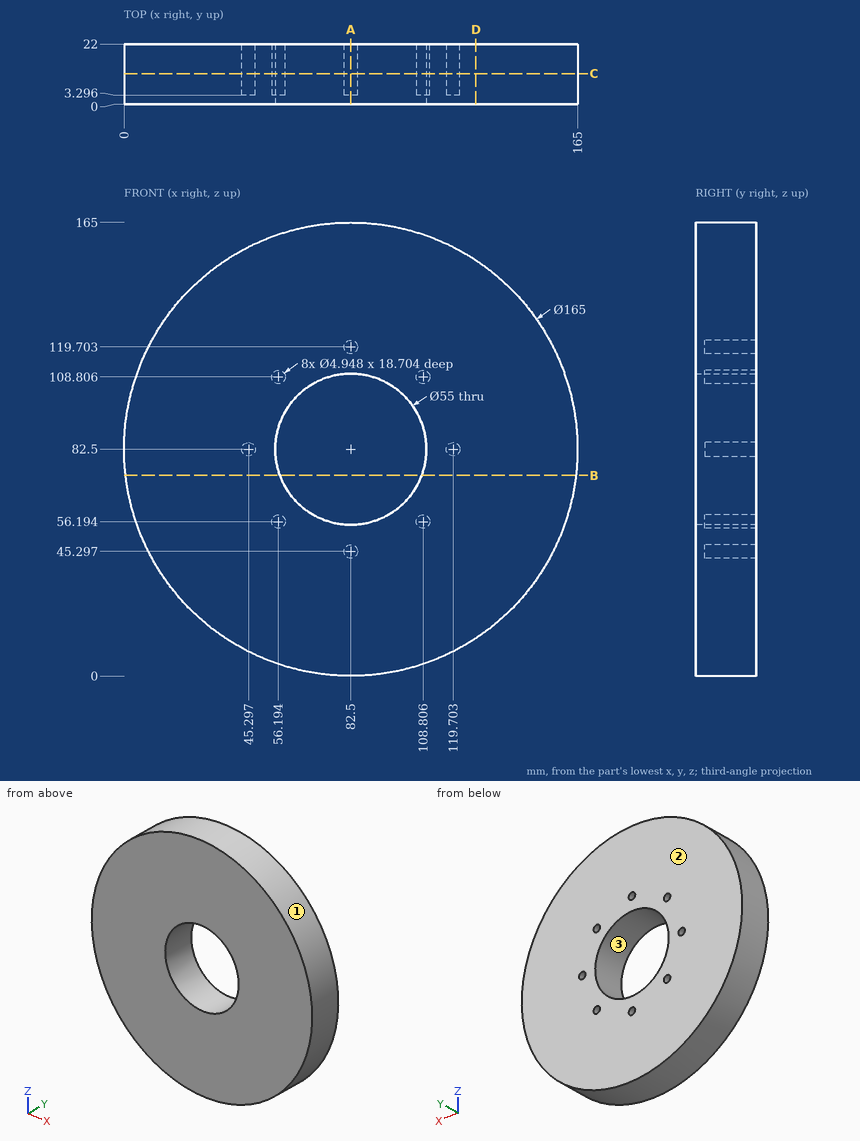
Answer from the drawing. Dimensions are ordinates in mm from the lowest x, y and z of the part. Give positions to 0.01 mm unless a question says otherwise; leave off trailing zeros. Write each loop counter-clockwise with the first axis right and the second up, starting at its lowest first coordinate (ties: lowest second). Pieces come first, ordered by that corner, then holes. Notation, with made-up numbers: (23.5, -32) -> (45.5, -32) arc R26 ccw to (45.5, -10) -> close; hole circle Ø3 at (19.25, 66). An arc over 180 degrees is marked (long way). Use a Markdown table: item, result.
(1) Flat-ended cylindrical pins translate along their axes: P1, Ø12, axis at y = 7.5, z = 147, coming from the -X side; P2, Ø1.5, axis at y = 3, z = 143.5, coming from the -X side; P3, Ø1, axis at y = 6, z = 104, coming from the -X side. Find the tip coordinate at first contact, or state that the pin passes through.
Return value:
| item | result |
|---|---|
| P1 | x = 24.33 |
| P2 | x = 26.14 |
| P3 | x = 2.72 |
(2) Find the intervals of material crossed by probe 1 along X at (y, z) = (11.25, 82.5); probe 2 along Z at (x, y) = (75.5, 16.5) (1 decimal); probe 3 along Z at (x, y) = (96, 13.5), in increasing order. Write a range as from..to.
Return value:
| item | result |
|---|---|
| probe 1 | 0..42.82, 47.77..55, 110..117.23, 122.18..165 |
| probe 2 | 0.3..55.9, 109.1..164.7 |
| probe 3 | 1.11..58.54, 106.46..163.89 |
(3) Section C-C, the plane y = 11.25 is taken. Give the number of separate pieces and of enclosed holes in the cut face, then the cut area to 3 significant figures.
Return value:
| item | result |
|---|---|
| separate pieces | 1 |
| enclosed holes | 9 |
| area | 18,900 mm2 |
(4) Section B-B, the plane z = 73 is taken. Determine the outline of the cut face in (x, y).
Return value:
| item | result |
|---|---|
| outline | (0.55, 0) -> (56.69, 0) -> (56.69, 22) -> (0.55, 22) -> close; (108.31, 0) -> (164.45, 0) -> (164.45, 22) -> (108.31, 22) -> close |
(5) Determine the mould class of the marked faces 1, 2 and 3 for opening direction X: released by +X, released by -X, zero draft, split by the parting line, or undercut.
Return value:
| item | result |
|---|---|
| face 1 | split by the parting line |
| face 2 | zero draft |
| face 3 | undercut |
(6) Section A-A, the plane x = 82.5 is taken. Determine the outline of the cut face in (y, z).
Return value:
| item | result |
|---|---|
| outline | (0, 0) -> (22, 0) -> (22, 42.82) -> (3.3, 42.82) -> (3.3, 47.77) -> (22, 47.77) -> (22, 55) -> (0, 55) -> close; (0, 110) -> (22, 110) -> (22, 117.23) -> (3.3, 117.23) -> (3.3, 122.18) -> (22, 122.18) -> (22, 165) -> (0, 165) -> close |
(7) Section D-D, the plane x = 128 is taken. Determine the outline of the cut face in (y, z).
Return value:
| item | result |
|---|---|
| outline | (0, 13.68) -> (22, 13.68) -> (22, 151.32) -> (0, 151.32) -> close |
